from build123d import *

# Parameters (mm, degrees)
F0_R     = 15
F1_DEPTH = 150
F3_DEPTH = 120
F4_W     = 100
F4_H     = 1
F5_DEPTH = 1


with BuildPart() as f1:
    # F0 (on Right) → F1 (new body)
    with BuildSketch(Plane.YZ):
        Circle(F0_R)
    extrude(amount=F1_DEPTH)

    # F2 (on face) → F3 (cut)
    with BuildSketch(Plane.YZ.offset(150)):
        with BuildLine():
            ThreePointArc((15, 0), (0, 15), (-15, 0))
            Line((-15, 0), (15, 0))
        make_face()
    extrude(amount=-F3_DEPTH, mode=Mode.SUBTRACT)

    # F4 (on face) → F5 (cut)
    with BuildSketch(Plane.XY):
        with Locations((90, 0)):
            Rectangle(F4_W, F4_H)
    extrude(amount=-F5_DEPTH, mode=Mode.SUBTRACT)


solid = f1.part
Model file for the job. Use its own axes, mm. A direction names the side the tool comes from. Give positions to 0.01 mm unless a question says otherwise; leave off trailing zeros. Loops run counter-clockwise (first coordinate to the right, second up) from the corner with the lowest first, then second, coordinate; pieces in that order, holes last.
1) Saw through at C-C (z = 11.5). Write the cut outline in (x, y), plus the area to 3 significant figures.
2) Saw through at D-D (z = -10.75). Write the cut outline in (x, y), plus the area to 3 significant figures.
3) Flat gauge pins, fed straight in: pin 1 Ø0.5 at (x, y) = (99.5, 0) entering from +Z; pin 2 Ø12 at (x, y) = (128.5, -6.5) entering from -Z; pin 3 Ø10 at (x, y) = (57, 6.5) entering from -Z. Where does each tip first touch, or does it go through?
4) Wall check: line 1 (X direction, y = -4.5, z = 13.25); line 2 (Y direction, x = 46, z = -9); line 3 (Y direction, x = 27.5, z = 9.25). Give the ranges that are in metal, low to high.
5) Saw through at B-B (y = -3). Write the cut outline in (x, z), plus the area to 3 significant figures.
6) Tool access for faces 1 (the flat face through (0, 0, 0)), 2 (the flat face through (30, 0, 6)): list every direction of +Z, -Z, +X, -X, +Y, -Y with a clear straight run to the whole face (end or side of a thin tool).
7) Saw through at A-A (x = 121). Write the cut outline in (y, z).
Answer block:
1. outline: (0, -9.63) - (30, -9.63) - (30, 9.63) - (0, 9.63) - close
1. area: 578 mm2
2. outline: (0, -10.46) - (150, -10.46) - (150, 10.46) - (0, 10.46) - close
2. area: 3,140 mm2
3. pin 1: stops at z = -1
3. pin 2: stops at z = -14.99
3. pin 3: stops at z = -14.92
4. line 1: x = 0 to 30
4. line 2: y = -12 to 12
4. line 3: y = -11.81 to 11.81
5. outline: (0, -14.7) - (150, -14.7) - (150, 0) - (30, 0) - (30, 14.7) - (0, 14.7) - close
5. area: 2,650 mm2
6. face 1: +Z, -Z, -X, +Y, -Y
6. face 2: +Z, +X, +Y, -Y
7. outline: (-15, 0) arc R15 ccw to (15, 0) - (0.5, 0) - (0.5, -1) - (-0.5, -1) - (-0.5, 0) - close
